Autodesk Inventor part; units mm, degrees
ref_plane "Work Plane1" through (-16.8587, 0, 0) normal (0, -0.866, -0.5) x (1, 0, 0)
ref_plane "YZ Plane" through (0, 0, 0) normal (1, 0, 0) x (0, 1, 0)
ref_plane "XZ Plane" through (0, 0, 0) normal (0, 1, 0) x (-1, 0, 0)
sketch "Sketch1" plane through (0, 0, 0) normal (1, 0, 0) x (0, 1, 0)
  line L0 (-9.2376, 0) -> (-4.6188, 8)
  line L1 (-4.6188, 8) -> (4.6188, 8)
  line L2 (4.6188, 8) -> (9.2376, 0)
  line L3 (9.2376, 0) -> (4.6188, -8)
  line L4 (4.6188, -8) -> (-4.6188, -8)
  line L5 (-4.6188, -8) -> (-9.2376, 0)
  point P0 (0, 0)
  point P1 (0, 0)
  dimension "d0" = 18.4752
extrude "Body" add sketch "Sketch1" along normal blind 9.5
sketch "Sketch2" plane through (0, 0, 0) normal (0, 0, 1) x (1, 0, 0)
  line L0 (0, 4.6188) -> (0, 9.2376)
  line L1 (0, 9.2376) -> (9.5, 9.2376)
  line L2 (9.5, 4.6188) -> (9.5, 9.2376)
  line L3 (-1.9, 0) -> (11.4, 0)
  line L4 (1.1475, 9.2376) -> (0, 7.25)
  line L5 (8.3525, 9.2376) -> (9.5, 7.25)
  dimension "d3" = 30
  dimension "d4" = 30
  dimension "d5" = 14.5
  dimension "d6" = 14.5
revolve "Chamfer1" cut sketch "Sketch2" angle 360 about axis through (-10, 0, 0) along (1, 0, 0)
sketch "Sketch3" plane through (9.5, 0, 0) normal (1, 0, 0) x (0, 0, -1)
  arc A0 (-0.625, -1.0825) -> (0.625, -1.0825) centre (0, 0) ccw
hole "Thread" at (9.5, 0, 0) direction (-1, 0, 0) diameter 8.376 end through all
chamfer "Chamfer2" distance 0.8119 angle 30 1 edges at (9.5, 0, 4.188) measured on face at (9.5, 6.1489, -0.7466)
chamfer "Chamfer3" distance 0.8119 angle 30 1 edges at (0, 0, 4.188) measured on face at (0, 6.1489, -0.7466)
ref_plane "Work Plane1" through (-16.8587, 0, 0) normal (0, -0.866, -0.5) x (1, 0, 0)
equation "\"d0\" = 1.1547 * SW"
equation "\"d1\" = KOH"
equation "\"d3\" = ANG1"
equation "\"d4\" = ANG2"
equation "\"d5\" = SW0"
equation "\"d6\" = SW01"
equation "\"d8\" = -0.5 * GD1 + 0.5 * NND"
equation "\"d40\" = -0.5 * GD1 + 0.5 * NND"
equation "\"d10\" = -0.5 * GD1 + 0.5 * NND"
equation "\"d41\" = -0.5 * GD1 + 0.5 * NND"
equation "\"ANG1\" = 30deg"
equation "\"ANG2\" = 30deg"
equation "\"KOH\" = 9.5"
equation "\"SW\" = 16"
equation "\"SW0\" = 14.5"
equation "\"SW01\" = 14.5"
equation "\"GUL\" = 0.541266 * PTC"
equation "\"TOA\" = 30deg"
equation "\"PTC\" = 1.5"
equation "\"E0\" = 1.155 * SW"
equation "\"GAL\" = 0.541266 * PTC"
properties part number "ISO 4034 - M10" material "Stainless Steel"
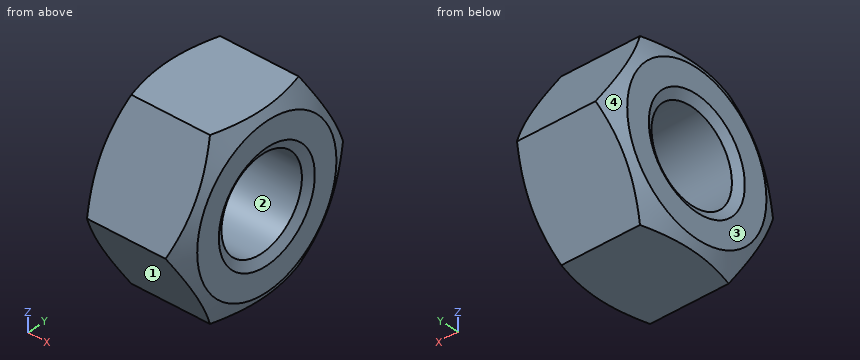
The listing builds one solid part. Answer for the finished solid, in the listing's coordinates (mm). Face numbers are marked on the shaded views. Round coordinates to 2 decimals unless told otherwise and drop trailing zeros. Write each loop counter-clockwise with the first axis right and the second up, starting at its lowest first coordinate (ties: lowest second). Pieces come first, ordered by that corner, then holes. Notation, with made-up numbers: (55.5, 71) - (64.5, 71) arc R19 cw to (64.5, 99) - close; hole circle Ø2 at (-24, 53.25). An arc over 180 degrees is marked (long way). Use one line per item in the form item = value. Start each with the question number.
Item 1: A cutting plane is placed at A-A (y = 0). Write down the section's boundary in (x, z).
Item 2: Find the intervals of material crossed by line 1 (Z direction, x = 5, y = 0); line 2 (Y direction, x = 0.5, z = 2.25); line 3 (Z direction, x = 2.25, y = 1.75), in increasing order. Write a range as [from, to].
Item 3: Flat-ended cylindrical pins translate along their axes: pin 1 Ø1.5 at (x, z) = (8, 3) entering from +Y; pin 2 Ø5 at (y, z) = (-4, -1.5) entering from +X; pin 3 Ø3 at (x, z) = (1.5, -4.5) entering from -Y. Find the tip coordinate at first contact, or state that the pin passes through.
Item 4: Determine the mould class of the marked faces 1, 2, 3 and 4 for opening direction Y: +Y half, -Y half, draft (parallel to the pull), parting line (faces both ways), or undercut.
Item 5: A cutting plane is placed at B-B (x = 3.5). Write down the section's boundary in (y, z), plus the area to 3 significant figures.
The answers:
q1.outline = (0, -7.25) - (0.43, -8) - (9.07, -8) - (9.5, -7.25) - (9.5, -5) - (9.03, -4.19) - (0.47, -4.19) - (0, -5) - close; (0, 5) - (0.47, 4.19) - (9.03, 4.19) - (9.5, 5) - (9.5, 7.25) - (9.07, 8) - (0.43, 8) - (0, 7.25) - close
q2.line_1 = [-8, -4.19], [4.19, 8]
q2.line_2 = [-7.8, -3.53], [3.53, 7.8]
q2.line_3 = [-8, -3.8], [3.8, 8]
q3.pin_1 = 7.94
q3.pin_2 = 9.5
q3.pin_3 = -7.51
q4.face_1 = -Y half
q4.face_2 = undercut
q4.face_3 = draft
q4.face_4 = parting line
q5.outline = (-9.24, 0) - (-4.62, -8) - (4.62, -8) - (9.24, 0) - (4.62, 8) - (-4.62, 8) - close; hole circle Ø8.38 at (0, 0)
q5.area = 167 mm^2
